Source: CAD feature listing. Evaluate the final solid. Frame: model axes, mm. Coordinates: 2 decimals unless noted, no trailing zeros. Order: outer loops, then holes, each group sorted by start corner. A loop starts at its lowest first (then second) coordinate and runs counter-clockwise, first axis right, second up. Notation, with made-up numbers: (0.5, 54.25) -> (7.5, 54.25) arc R28 cw to (7.5, 81.25) -> close; hole circle Ø2 at (85, 55). An arc over 180 degrees is marked (long way). Put each result on its own line as item: value.
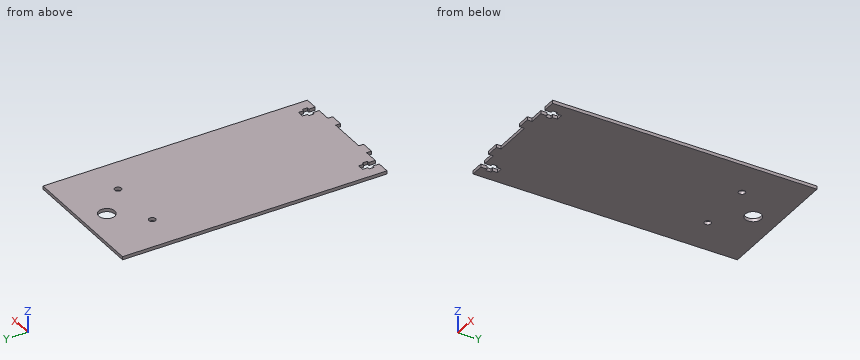
from build123d import *

# Parameters (mm, degrees)
SKETCH_1_R      = 5.05
SKETCH_1_R_2    = 2.05
EXTRUDE_1_DEPTH = 2


with BuildPart() as part:
    # 草图1 → 凸台-拉伸1 (new body)
    with BuildSketch(Plane.XY):
        Polygon((-28.741188564, 3.13029316), (-28.741188564, 7.13029316), (-27.291188564, 7.13029316), (-27.291188564, 10.33029316), (-28.741188564, 10.33029316), (-28.741188564, 13.53029316), (-32.841188564, 13.53029316), (-32.841188564, 10.33029316), (-34.291188564, 10.33029316), (-34.291188564, 7.13029316), (-32.841188564, 7.13029316), (-32.841188564, 3.13029316), (-40.841188564, 3.13029316), (-40.841188564, 168.13029316), (41.258811436, 168.13029316), (41.258811436, 3.13029316), (33.258811436, 3.13029316), (33.258811436, 7.13029316), (34.708811436, 7.13029316), (34.708811436, 10.33029316), (33.258811436, 10.33029316), (33.258811436, 13.53029316), (29.158811436, 13.53029316), (29.158811436, 10.33029316), (27.708811436, 10.33029316), (27.708811436, 7.13029316), (29.158811436, 7.13029316), (29.158811436, 3.13029316), (20.208811436, 3.13029316), (20.208811436, 0.13029316), (12.208811436, 0.13029316), (12.208811436, 3.13029316), (-11.791188564, 3.13029316), (-11.791188564, 0.13029316), (-19.791188564, 0.13029316), (-19.791188564, 3.13029316), align=None)
        with Locations((0.208811436, 153.13029316)):
            Circle(SKETCH_1_R, mode=Mode.SUBTRACT)
        with Locations((17.886480965, 135.45262363)):
            Circle(SKETCH_1_R_2, mode=Mode.SUBTRACT)
        with Locations(Location((-17.468858094, 135.45262363, 0), (0, 0, 180))):
            Circle(SKETCH_1_R_2, mode=Mode.SUBTRACT)
    extrude(amount=EXTRUDE_1_DEPTH)


solid = part.part
1. Cut plane A-A on x = -17.5. Output: boundary loops of the cut face in (y, z), plus the area to 3 significant figures.
Numbers:
outline: (0.13, 0) -> (133.4, 0) -> (133.4, 2) -> (0.13, 2) -> close; (137.5, 0) -> (168.13, 0) -> (168.13, 2) -> (137.5, 2) -> close
area: 328 mm2
2. First-contact query: pin 1 (1 mm diameter, centred on y = 1, z = 1.5, fed in from -X); pin 2 (1.2 mm diameter, centred on x = -27.5, z = 1, fed in from -Y). Flat tips, straight axial feed; report the tip coordinate or a pass-through.
Numbers:
pin 1: stops at x = -19.79
pin 2: stops at y = 3.13
3. Ray query, line 1 along X through (y, z) = (10, 1.05); line 2 along Y through (x, z) = (-34, 0.7); line 3 along Y through (x, z) = (-20, 1.15). Return the intervals inside material, ascending.
Numbers:
line 1: x = -40.84 to -34.29, -27.29 to 27.71, 34.71 to 41.26
line 2: y = 3.13 to 7.13, 10.33 to 168.13
line 3: y = 3.13 to 168.13
4. Cut plane B-B on z = 0.9. Count the separate pieces of the cut face and the enclosed holes in it, plus the area to 3 significant figures.
Numbers:
separate pieces: 1
enclosed holes: 3
area: 13,400 mm2
